Input: part model. Units: mm. Frame: model coordinates. A direction names the side the tool comes from. Coordinates: 2 decimals unless noted, no trailing zeros. Write each loop counter-clockwise with the first axis right and the second up, starting at its lowest first coordinate (ties: lowest second). Pieces come first, ordered by that corner, then holes.
1) Section query A-A (y = -12.7). Output: boundary loops of the cut face in (x, z), then the cut area to 3 significant figures.
2) Section query C-C (y = -3). Output: boundary loops of the cut face in (x, z).
3) Set-up query: faces 4 (the cylindrical face through (14.789, 18.872, -1.703)), 5 (the cylindrical face through (1.402, 0.893, -16.246)), 6 (the cylindrical face through (12.52, -9.36, 10.6)). Return all of +Z, -Z, +X, -X, +Y, -Y with unobstructed straight access to the full face (end or side cutting, diameter ignored); none if empty.
4) Pin query (flat end, axial travel): pin 1 Ø20 at (y, z) = (-12.7, 0) entering from +X (3 decimals); pin 2 Ø3.5 at (y, z) = (-26.17, 13.47) entering from -X. Return the tip coordinate at first contact, or that it passes through.
5) Line query: L1, parallel to Y at x = 15.5, z = -13; L2, parallel to Z at x = 2, y = -26; L3, parallel to Y at x = 4.5, z = -8.5. Output: solid intervals per line, ascending.
6) Section query B-B (x = 12.7). State how many separate pieces and enclosed holes the cut face has, then the cut area to 3 significant figures.
7) Draft query along X for faces 1 (the flat face through (13, 31.75, 0)), 2 (the flat face through (2.845, -25, 12)), 3 (the cylindrical face through (16.313, 18.872, 17.846)). Return one class per face: pulls with the +X half, pulls with the -X half, needs draft (parallel to the pull), parting line crosses it, or undercut.
from build123d import *

# Parameters (mm, degrees)
SKETCH1_W                                      = 50.8
SKETCH1_H                                      = 63.5
BASE_DEPTH                                     = 25.4
F_7_8_0_875_DIAMETER_HOLE1_D                   = 22.225
F_10_32_TAPPED_HOLE1_D                         = 4.0386
F_10_32_TAPPED_HOLE1_DEPTH                     = 25.4
F_10_32_TAPPED_HOLE1_TIP                       = 1.213317848
CBORE_FOR_4_SOCKET_HEAD_CAP_SCREW1_D           = 3.2639
CBORE_FOR_4_SOCKET_HEAD_CAP_SCREW1_CBORE_D     = 5.55752
CBORE_FOR_4_SOCKET_HEAD_CAP_SCREW1_CBORE_DEPTH = 2.8448
CIRPATTERN1_COUNT                              = 4
CHAMFER2_SIZE                                  = 6.35
F_10_32_TAPPED_HOLE2_D                         = 4.0386


with BuildPart() as part:
    # Sketch1 → Base (new body)
    with BuildSketch(Plane(origin=(0, 0, 0), x_dir=(0, 0, -1), z_dir=(1, 0, 0))):
        Rectangle(SKETCH1_W, SKETCH1_H)
    extrude(amount=BASE_DEPTH)

    # 7/8 (0.875) Diameter Hole1 (through all)
    with Locations(Plane(origin=(25.4, 0, 0), x_dir=(0, 0, -1), z_dir=(1, 0, 0))):
        with Locations((0, -12.7)):
            Hole(F_7_8_0_875_DIAMETER_HOLE1_D / 2)

    # #10-32 Tapped Hole1
    with Locations(Plane(origin=(0, 31.75, 0), x_dir=(1, 0, 0), z_dir=(0, 1, 0))):
        with Locations((15.875, 15.875), (15.875, -15.875), (15.875, 0)):
            Hole(F_10_32_TAPPED_HOLE1_D / 2, depth=F_10_32_TAPPED_HOLE1_DEPTH)
            with Locations((0, 0, -(F_10_32_TAPPED_HOLE1_DEPTH + F_10_32_TAPPED_HOLE1_TIP / 2))):  # 118° drill point
                Cone(0, F_10_32_TAPPED_HOLE1_D / 2, F_10_32_TAPPED_HOLE1_TIP, mode=Mode.SUBTRACT)

    # CBORE for #4 Socket Head Cap Screw1 (through all)
    with Locations(Plane.ZY):
        with Locations((-13.470384182, 0.770384182)):
            cbore_for_4_socket_head_cap_screw1 = CounterBoreHole(CBORE_FOR_4_SOCKET_HEAD_CAP_SCREW1_D / 2, CBORE_FOR_4_SOCKET_HEAD_CAP_SCREW1_CBORE_D / 2, CBORE_FOR_4_SOCKET_HEAD_CAP_SCREW1_CBORE_DEPTH)

    # CirPattern1: CBORE for #4 Socket Head Cap Screw1 ×4 about axis
    cirpattern1_axis = Axis((0, -12.7, 0), (1, 0, 0))
    for i in range(1, CIRPATTERN1_COUNT):
        add(cbore_for_4_socket_head_cap_screw1.rotate(cirpattern1_axis, i * 360 / CIRPATTERN1_COUNT), mode=Mode.SUBTRACT)

    # Chamfer2
    chamfer2_edges = [part.edges().sort_by_distance(p)[0] for p in [
        (12.7, -31.75, -25.4),
        (12.7, -31.75, 25.4),
    ]]
    chamfer(chamfer2_edges, length=CHAMFER2_SIZE)

    # #10-32 Tapped Hole2 (through all)
    with Locations(Plane(origin=(0, 0, -25.4), x_dir=(-1, 0, 0), z_dir=(0, 0, -1))):
        with Locations((-12.7, -12.7)):
            Hole(F_10_32_TAPPED_HOLE2_D / 2)


solid = part.part
Answer:
1. outline: (0, -25.4) - (10.68, -25.4) - (10.68, -11.11) - (0, -11.11) - close; (0, 11.11) - (10.68, 11.11) - (10.68, 25.4) - (0, 25.4) - close; (14.72, -25.4) - (25.4, -25.4) - (25.4, -11.11) - (14.72, -11.11) - close; (14.72, 11.11) - (25.4, 11.11) - (25.4, 25.4) - (14.72, 25.4) - close
1. area: 610 mm2
2. outline: (0, -25.4) - (25.4, -25.4) - (25.4, -5.42) - (0, -5.42) - close; (0, 5.42) - (25.4, 5.42) - (25.4, 25.4) - (0, 25.4) - close
3. face 4: +Y
3. face 5: -X
3. face 6: +X, -X
4. pin 1: passes through
4. pin 2: stops at x = 2.84
5. L1: y = -31.75 to -27.73, -24.61 to -0.79, 2.33 to 31.75
5. L2: z = -24.8 to -16.24, -10.7 to 10.7, 16.24 to 24.8
5. L3: y = -31.75 to -19.86, -5.54 to 31.75
6. separate pieces: 2
6. enclosed holes: 4
6. area: 2,650 mm2
7. face 1: needs draft
7. face 2: pulls with the -X half
7. face 3: undercut
